CAD build for the part. Positions are in the model's coordinates, mm. A direction names the side the tool comes from. Coordinates: 2 decimals unless noted, no trailing zeros. Write each loop counter-clockwise with the first axis right and the second up, starting at its lowest first coordinate (ties: lowest second). Pieces come first, ordered by that corner, then holes. Notation, with made-up numbers: (69.5, 63.5) - (101.5, 63.5) arc R16 cw to (101.5, 67.5) - close; hole circle Ø8 at (6, -11.75). An arc over 180 degrees is marked (long way). One line per question, with ' | ' between items. Start each with the question number.
1. Band-saw the part on D-D, the plane x = 10.25. Write the cut outline in (y, z), then the cut area to 3 significant figures.
2. Band-saw the part on B-B, the plane x = 2.25. Write the cut outline in (y, z).
3. Band-saw the part on C-C, the plane y = 0.5. Write the cut outline in (x, z).
4. Probe line 1 (Y direction, x = 20.25, z = -8); line 2 (X direction, y = 2.55, z = -9); line 3 (X direction, y = 0.8, z = -7.75). List the from-to ranges inside material, lowest first.
5. Two-plate mould, pull along Y, no slides. Class faces 4 (the flat face through (10.9, 0.5, 0)), 5 (the flat face through (2, 3.2, -9)), 6 (the flat face through (1.54, 1.88, -11.6)): +Y half, -Y half, draft (parallel to the pull), parting line (faces both ways), or undercut.
6. Which spindle directions (+Z, -Z, +X, -X, +Y, -Y) get a long thin tool onto all of the face, cutting with end or side? Do faces 1 (the flat face through (-1.2, 2, -9)), 2 (the flat face through (-1, 1, -8)), 3 (the flat face through (4.2, 2, -9)). Say none if no direction does.
7. Flat gauge pins, fed straight in: P1, Ø0.6, axis at y = 1, z = -5, coming from the -X side; P2, Ø3, axis at x = 11, z = -2, coming from the +Y side; P3, Ø1.3, axis at x = -1, z = -9, coming from the -Y side. Where does each tip first touch, or does it go through?
8. Band-saw the part on A-A, the plane z = -9.25. Write the cut outline in (x, y).
Autodesk Fusion 360 part; units mm, degrees
sketch "Sketch1" plane through (0, 0, 0) normal (0, 1, 0) x (1, 0, 0)
  line L0 (0, 0) -> (22.2, 0)
  line L1 (22.2, 0) -> (22.2, 17)
  line L2 (22.2, 17) -> (0, 17)
  line L3 (0, 17) -> (0, 0)
  dimension "d1" = 22.2
  dimension "d2" = 17
extrude "Extrude1" add sketch "Sketch1" along normal blind 1
sketch "Sketch2" plane through (0, 0, 0) normal (-1, 0, 0) x (0, 0, 1)
  line L0 (-17, 0) -> (0, 0)
  line L1 (0, 0) -> (0, 1)
  line L2 (0, 1) -> (-17, 1)
  line L3 (-17, 1) -> (-17, 0)
  line L4 (-12.2, 3.2) -> (-4.8, 3.2)
  line L5 (-4.8, 3.2) -> (-5.7974, 1)
  line L6 (-11.1974, 1) -> (-12.2, 3.2)
  point P0 (-8.5, 1)
  point P1 (-8.5, 3.2)
  dimension "d5" = 7.4
  dimension "d6" = 5.4
  dimension "d7" = 2.2
  dimension "d8" = 114.5
extrude "Extrude2" add sketch "Sketch2" along normal blind 1.2 and the other way blind 4.2 contours L2 L4 L5 L6
fillet "Fillet1" radius 0.3 4 edges at (1.5, 3.2, -4.8) (1.5, 3.2, -12.2) (-0.6, 1, -5.7974) (-0.6, 1, -11.1974)
Filled in:
1) outline: (0, -17) - (1, -17) - (1, 0) - (0, 0) - close | area: 17.0 mm²
2) outline: (0, -17) - (1, -17) - (1, -11.2) - (2.78, -12.01) arc R0.3 ccw to (3.2, -11.73) - (3.2, -5.27) arc R0.3 ccw to (2.78, -4.99) - (1, -5.8) - (1, 0) - (0, 0) - close
3) outline: (0, -17) - (22.2, -17) - (22.2, 0) - (0, 0) - close
4) line 1: y = 0 to 1 | line 2: x = -1.2 to 4.2 | line 3: x = 0 to 22.2
5) face 4: draft | face 5: +Y half | face 6: undercut
6) face 1: +Z, -Z, -X, +Y, -Y | face 2: +Z, -Z, -X, -Y | face 3: +Z, -Z, +X, +Y
7) P1: stops at x = 0 | P2: stops at y = 1 | P3: stops at y = 1
8) outline: (-1.2, 1) - (0, 1) - (0, 0) - (22.2, 0) - (22.2, 1) - (4.2, 1) - (4.2, 3.2) - (-1.2, 3.2) - close
